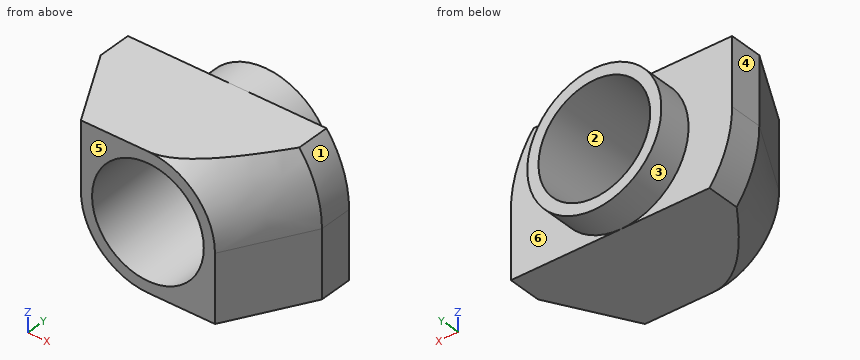
from build123d import *

# Parameters (mm, degrees)
EXTRUDE_1_DEPTH       = 3
HOLE_WIZARD_M61_D     = 5
HOLE_WIZARD_M61_DEPTH = 6.5
SKETCH_4_OUTSIDE_W    = 14.556
SKETCH_4_OUTSIDE_H    = 10.656
SKETCH_4_OUTSIDE_R    = 3
CUT_EXTRUDE_1_DEPTH   = 1.5
CUT_EXTRUDE_2_DEPTH   = 6


with BuildPart() as part:
    # Эскиз1 → Бобышка-Вытянуть1 (new body, symmetric)
    with BuildSketch(Plane.XY):
        Polygon((3, 0), (-3, 0), (-3, -1.5), (-4.95, -1.5), (-4.95, -6.5), (4.95, -6.5), (4.95, -1.5), (3, -1.5), align=None)
    extrude(amount=EXTRUDE_1_DEPTH, both=True)

    # Отверстие обработанное метчиком M61
    with Locations(Plane(origin=(0, 0, 0), x_dir=(1, 0, 0), z_dir=(0, 1, 0))):
        with Locations((0, 0)):
            Hole(HOLE_WIZARD_M61_D / 2, depth=HOLE_WIZARD_M61_DEPTH)

    # Эскиз4 outside → Вырез-Вытянуть1 (cut)
    with BuildSketch(Plane(origin=(0, 0, 0), x_dir=(1, 0, 0), z_dir=(0, 1, 0))):
        Rectangle(SKETCH_4_OUTSIDE_W, SKETCH_4_OUTSIDE_H)
        with Locations(Location((0, 0, 0), (0, 0, 270))):  # turned: the seam where the file's is
            Circle(SKETCH_4_OUTSIDE_R, mode=Mode.SUBTRACT)
    extrude(amount=-CUT_EXTRUDE_1_DEPTH, mode=Mode.SUBTRACT)

    # Эскиз5 → Вырез-Вытянуть2 (cut, through all)
    with BuildSketch(Plane(origin=(0, -1.5, 0), x_dir=(1, 0, 0), z_dir=(0, 1, 0))):
        with BuildLine():
            Line((-4.95, 0), (-4.95, 3))
            Line((-4.95, 3), (-3.937321425, 3))
            ThreePointArc((-3.937321425, 3), (-4.690002188, 1.583154912), (-4.95, 0))
        make_face()
        with BuildLine():
            Line((4.95, 0), (4.95, -3))
            Line((4.95, -3), (3.937321425, -3))
            ThreePointArc((3.937321425, -3), (4.690002188, -1.583154912), (4.95, 0))
        make_face()
    extrude(amount=-CUT_EXTRUDE_2_DEPTH, mode=Mode.SUBTRACT)

    # Вырез-По траектории1: sweep along a path in Эскиз7
    with BuildLine(Plane.XZ.offset(6.5)) as sweep_1_path:
        Line((0, 4.95), (-4.95, 4.95))
        Line((-4.95, 4.95), (-4.95, 0))
        ThreePointArc((-4.95, 0), (-3.500178567, -3.500178567), (0, -4.95))
        Line((0, -4.95), (4.95, -4.95))
        Line((4.95, -4.95), (4.95, 0))
        ThreePointArc((4.95, 0), (3.500178567, 3.500178567), (0, 4.95))
    # Эскиз6 → Вырез-По траектории1 (sweep, cut)
    with BuildSketch(Plane.XY.offset(3)):
        Polygon((-4.95, -3), (-4.95, -6.5), (-3, -6.5), align=None)
    sweep(path=sweep_1_path.line, transition=Transition.RIGHT, mode=Mode.SUBTRACT)


solid = part.part
Work out the finished part from the listing and answer in its coordinate system (mm). Face numbers are marked on the shaded views. A direction names the side the tool comes from. Give positions to 0.01 mm unless a question says otherwise; leave off trailing zeros. Write each loop counter-clockwise with the first axis right and the second up, starting at its lowest first coordinate (ties: lowest second). Pieces come first, ordered by that corner, then holes.
Q1. The part is cut by section B-B on y = -4.25. Give the vertices of the cut face in (x, z), and give its area (3 significant figures).
Answer:
outline: (-4.25, 0) arc R4.25 ccw to (-3.02, -3) - (4.25, -3) - (4.25, 0) arc R4.25 ccw to (3.02, 3) - (-4.25, 3) - close; hole circle Ø5 at (0, 0)
area: 29.1 mm2
Q2. The part is cut by section C-C on y = -0.75. Give the vertices of the cut face in (x, z), and give its area (3 significant figures).
Answer:
outline: circle Ø6 at (0, 0); hole circle Ø5 at (0, 0)
area: 8.64 mm2
Q3. For a pull along Z with two mould halves and no side action, classify the marked faces 1, 2, 3 and 4 as released by +Z, released by -Z, zero draft, split by the parting line, or undercut.
Answer:
face 1: released by +Z
face 2: undercut
face 3: split by the parting line
face 4: zero draft
Q4. A tool of negligible diameter and unlimited length cuts with its end or side. For the marked faces 5 and 6, from which of +Z, -Z, +X, -X, +Y, -Y can it reach the whole face along a straight path? Write none if from no direction.
Answer:
face 5: +Z, -Z, +X, -X, -Y
face 6: +X, +Y
Q5. Straight lines are drawn through the part: L1, parallel to Z at x = 0, y = -2.75; L2, parallel to X at y = -2.25, z = -2; L3, parallel to Z at x = -0.5, y = -4. For each, find the intervals that lie inside material, in ascending order.
Answer:
L1: z = -3 to -2.5, 2.5 to 3
L2: x = -4.53 to -1.5, 1.5 to 4.95
L3: z = -3 to -2.45, 2.45 to 3
Q6. The part is cut by section A-A on y = -5.75. Give the vertices of the cut face in (x, z), and give its area (3 significant figures).
Answer:
outline: (-3.42, 0) arc R3.42 ccw to (-1.64, -3) - (3.42, -3) - (3.42, 0) arc R3.42 ccw to (1.64, 3) - (-3.42, 3) - close; hole circle Ø5 at (0, 0)
area: 18.3 mm2
